Can you work these out from the model? Positions are in its coordinate system, mm. Coordinates: 2 decimals unless noted, no trailing zeros. Loops run counter-clockwise (first coordinate to the right, second up) from the corner with the lowest first, then second, coordinate; pieces in that order, holes last. Notation, with made-up numbers: M 21.25,53.5 L 27.25,53.5 A23 cw 27.25,82.5 Z; hole C 44,4.5 d5. An arc over 180 degrees is marked long. Return JSON: item names as keys, results as strings. Group by question number.
```python
from build123d import *

# Parameters (mm, degrees)
SKETCH1_W           = 177.8
SKETCH1_H           = 67.31
BOSS_EXTRUDE1_DEPTH = 3.175
CUT_EXTRUDE2_DEPTH  = 4.175
SKETCH5_W           = 127
SKETCH5_H           = 12.7
CUT_EXTRUDE3_DEPTH  = 4.175
SKETCH7_W           = 25.4
SKETCH7_H           = 38.1
BOSS_EXTRUDE2_DEPTH = 3.175
CUT_EXTRUDE4_DEPTH  = 4.175
FILLET3_R           = 5.08
SKETCH9_W           = 6.35
SKETCH9_H           = 92.71
CUT_EXTRUDE5_DEPTH  = 4.175
FILLET4_R           = 2.54
FILLET5_R           = 5.08
SKETCH10_W          = 146.05
SKETCH10_H          = 36.83
CUT_EXTRUDE6_DEPTH  = 4.175
FILLET6_R           = 2.54


with BuildPart() as part:
    # Sketch1 → Boss-Extrude1 (new body)
    with BuildSketch(Plane(origin=(0, 0, 0), x_dir=(1, 0, 0), z_dir=(0, 1, 0))):
        with Locations((88.9, 33.655)):
            Rectangle(SKETCH1_W, SKETCH1_H)
    extrude(amount=BOSS_EXTRUDE1_DEPTH)

    # Sketch4 → Cut-Extrude2 (cut, through all)
    with BuildSketch(Plane(origin=(0, 3.175, 0), x_dir=(1, 0, 0), z_dir=(0, 1, 0))):
        with BuildLine():
            Line((11.1125, 67.31), (11.1125, 62.23))
            ThreePointArc((11.1125, 62.23), (12.7, 60.6425), (14.2875, 62.23))
            Line((14.2875, 62.23), (14.2875, 67.31))
            Line((14.2875, 67.31), (11.1125, 67.31))
        make_face()
        with BuildLine():
            Line((166.6875, 67.31), (166.6875, 62.23))
            ThreePointArc((166.6875, 62.23), (165.1, 60.6425), (163.5125, 62.23))
            Line((163.5125, 62.23), (163.5125, 67.31))
            Line((163.5125, 67.31), (166.6875, 67.31))
        make_face()
    extrude(amount=-CUT_EXTRUDE2_DEPTH, mode=Mode.SUBTRACT)

    # Sketch5 → Cut-Extrude3 (cut, through all)
    with BuildSketch(Plane(origin=(0, 3.175, 0), x_dir=(1, 0, 0), z_dir=(0, 1, 0))):
        with Locations((88.9, 60.96)):
            Rectangle(SKETCH5_W, SKETCH5_H)
    extrude(amount=-CUT_EXTRUDE3_DEPTH, mode=Mode.SUBTRACT)

    # Sketch7 → Boss-Extrude2 (add)
    with BuildSketch(Plane(origin=(0, 3.175, 0), x_dir=(1, 0, 0), z_dir=(0, 1, 0))):
        with Locations((12.7, 73.66)):
            Rectangle(SKETCH7_W, SKETCH7_H)
        with Locations((165.1, 73.66)):
            Rectangle(SKETCH7_W, SKETCH7_H)
    extrude(amount=-BOSS_EXTRUDE2_DEPTH)

    # Sketch8 → Cut-Extrude4 (cut, through all)
    with BuildSketch(Plane(origin=(0, 3.175, 0), x_dir=(1, 0, 0), z_dir=(0, 1, 0))):
        with BuildLine():
            Line((11.1125, 92.71), (11.1125, 85.09))
            ThreePointArc((11.1125, 85.09), (12.7, 83.5025), (14.2875, 85.09))
            Line((14.2875, 85.09), (14.2875, 92.71))
            Line((14.2875, 92.71), (11.1125, 92.71))
        make_face()
        with BuildLine():
            Line((163.5125, 85.09), (163.5125, 92.71))
            Line((163.5125, 92.71), (166.6875, 92.71))
            Line((166.6875, 92.71), (166.6875, 85.09))
            ThreePointArc((166.6875, 85.09), (165.1, 83.5025), (163.5125, 85.09))
        make_face()
    extrude(amount=-CUT_EXTRUDE4_DEPTH, mode=Mode.SUBTRACT)

    # Fillet3
    fillet3_edges = [part.edges().sort_by_distance(p)[0] for p in [
        (25.4, 1.5875, -92.71),
        (0, 1.5875, -92.71),
        (177.8, 1.5875, -92.71),
        (152.4, 1.5875, -92.71),
    ]]
    fillet(fillet3_edges, radius=FILLET3_R)

    # Sketch9 → Cut-Extrude5 (cut, through all)
    with BuildSketch(Plane(origin=(0, 3.175, 0), x_dir=(1, 0, 0), z_dir=(0, 1, 0))):
        with Locations((3.175, 46.355)):
            Rectangle(SKETCH9_W, SKETCH9_H)
        with Locations((174.625, 46.355)):
            Rectangle(SKETCH9_W, SKETCH9_H)
    extrude(amount=-CUT_EXTRUDE5_DEPTH, mode=Mode.SUBTRACT)

    # Fillet4
    fillet4_edges = [part.edges().sort_by_distance(p)[0] for p in [
        (6.35, 1.5875, -92.71),
        (171.45, 1.5875, -92.71),
    ]]
    fillet(fillet4_edges, radius=FILLET4_R)

    # Fillet5
    fillet5_edges = [part.edges().sort_by_distance(p)[0] for p in [
        (6.35, 1.5875, 0),
        (171.45, 1.5875, 0),
    ]]
    fillet(fillet5_edges, radius=FILLET5_R)

    # Sketch10 → Cut-Extrude6 (cut, through all)
    with BuildSketch(Plane(origin=(0, 3.175, 0), x_dir=(1, 0, 0), z_dir=(0, 1, 0))):
        with Locations((88.9, 27.94)):
            Rectangle(SKETCH10_W, SKETCH10_H)
    extrude(amount=-CUT_EXTRUDE6_DEPTH, mode=Mode.SUBTRACT)

    # Fillet6
    fillet6_edges = [part.edges().sort_by_distance(p)[0] for p in [
        (15.875, 1.5875, -9.525),
        (15.875, 1.5875, -46.355),
        (161.925, 1.5875, -46.355),
        (161.925, 1.5875, -9.525),
    ]]
    fillet(fillet6_edges, radius=FILLET6_R)


solid = part.part
```
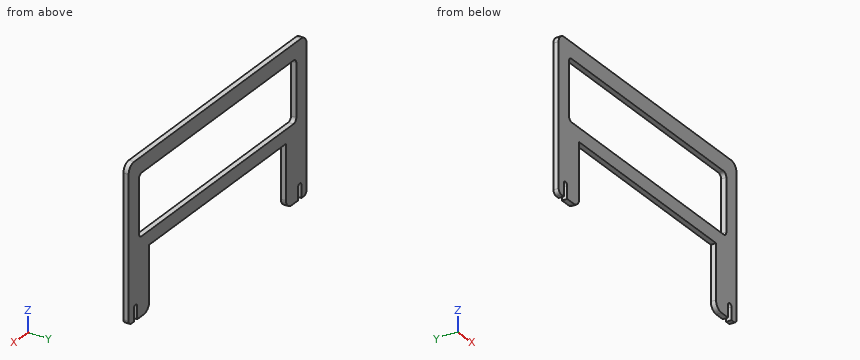
1) Suppose I cut it at C-C, the plane z = -40. List the corners of the cut face in (x, y) for me (3 decimals), then the cut area to 3 significant figures.
2) If I drill on line 1 (X direction, y = 2.95, z = -24) (3 decimals); line 2 (X direction, y = 2.6, z = -57); line 3 (Z direction, x = 101.5, y = 2.65) (3 decimals), over which ranges is the centre line in solid material (lowest first)? Write a range as from..to.
3) Suppose I cut it at A-A, the plane z = -58. List the corners of the cut face in (x, y) for me (3 decimals).
Returned:
{
 "1": {"outline": "M 6.35,0 L 15.875,0 L 15.875,3.175 L 6.35,3.175 Z; M 161.925,0 L 171.45,0 L 171.45,3.175 L 161.925,3.175 Z", "area": "60.5 mm²"},
 "2": {"line 1": "x = 6.35..15.875, 161.925..171.45", "line 2": "x = 6.35..25.4, 152.4..171.45", "line 3": "z = -54.61..-46.355, -9.525..0"},
 "3": {"outline": "M 6.35,0 L 25.4,0 L 25.4,3.175 L 6.35,3.175 Z; M 152.4,0 L 171.45,0 L 171.45,3.175 L 152.4,3.175 Z"}
}
